Design review of the part built by this model. Coordinates are the model's own, in mm. A direction names the side the tool comes from. Give positions to 0.01 mm unless a question says otherwise; leave off trailing zeros. Write each loop counter-clockwise with the first axis right and the second up, starting at its lowest first coordinate (ties: lowest second). Pieces come first, ordered by that corner, then holes. Notation, with made-up numbers: (-19, 12.5) -> (37, 12.5) arc R38 cw to (37, 50.5) -> close; hole circle Ø9 at (52.25, -13.75). An arc over 180 degrees is marked (long way). Answer as a JSON object with one key per item and string values.
```python
from build123d import *

# Parameters (mm, degrees)
SKETCH_R        = 55
PAD_DEPTH       = 40
PAD_DEPTH_BACK  = 20
POCKET_DEPTH    = 42
POCKET001_DEPTH = 16
SKETCH004_R     = 67.5
SKETCH004_R_2   = 58
POCKET002_DEPTH = 0.7
POCKET003_DEPTH = 0.7
SKETCH006_R     = 1.4
POCKET004_DEPTH = 35
SKETCH007_R     = 1.9
POCKET005_DEPTH = 20
FILLET_R        = 5
FILLET001_R     = 5
FILLET002_R     = 5
FILLET003_R     = 5
CHAMFER_SIZE    = 2
CHAMFER001_SIZE = 1


with BuildPart() as part:
    # Sketch → Pad (new body, two sides)
    with BuildSketch(Plane.XZ) as pad_sk:
        with BuildLine():
            Line((-120, 75), (0, 75))
            ThreePointArc((-74.66808, -7.048245), (55.468993, -50.479608), (0, 75))
            ThreePointArc((-74.66808, -7.048245), (-83.30852, 13.959176), (-102.203647, 26.566441))
            ThreePointArc((-120, 50.506104), (-115.063539, 35.591198), (-102.203647, 26.566441))
            Line((-120, 75), (-120, 50.506104))
        make_face()
        Circle(SKETCH_R, mode=Mode.SUBTRACT)
    extrude(amount=PAD_DEPTH)
    extrude(pad_sk.sketch, amount=-PAD_DEPTH_BACK)

    # Sketch001 (on Face7 of Pad) → Pocket (cut)
    with BuildSketch(Plane(origin=(0, 20, 0), x_dir=(1, 0, 0), z_dir=(0, 1, 0))):
        with BuildLine():
            Line((46.551104, -18.140074), (74.636799, -51.611301))
            ThreePointArc((74.636799, -51.611301), (27.033088, 86.623267), (-90.743475, 0))
            Line((-211.758942, -108.831918), (-90.743475, 0))
            Line((-62.856731, -108.831918), (-211.758942, -108.831918))
            Line((-42.167317, -48.745498), (-62.856731, -108.831918))
            Line((9.780971, -48.993879), (-42.167317, -48.745498))
            Line((46.551104, -18.140074), (9.780971, -48.993879))
        make_face()
    extrude(amount=-POCKET_DEPTH, mode=Mode.SUBTRACT)

    # Sketch003 (on Face2 of Pocket) → Pocket001 (cut)
    with BuildSketch(Plane(origin=(0, -22, 0), x_dir=(1, 0, 0), z_dir=(0, 1, 0))):
        with BuildLine():
            ThreePointArc((0, -70), (66.404243, -22.146705), (42.018147, 55.986385))
            Line((42.018147, 55.986385), (62.226624, 86.16832))
            Line((62.226624, 86.16832), (-170.809082, 86.16832))
            Line((-170.809082, 86.16832), (-170.809082, -70))
            Line((-170.809082, -70), (0, -70))
        make_face()
    extrude(amount=-POCKET001_DEPTH, mode=Mode.SUBTRACT)

    # Sketch004 → Pocket002 (cut)
    with BuildSketch(Plane(origin=(0, -38, 0), x_dir=(-1, 0, 0), z_dir=(0, 1, 0))):
        Circle(SKETCH004_R)
        Circle(SKETCH004_R_2, mode=Mode.SUBTRACT)
    extrude(amount=-POCKET002_DEPTH, mode=Mode.SUBTRACT)

    # Sketch005 (on Face14 of Pocket002) → Pocket003 (cut)
    with BuildSketch(Plane(origin=(0, -38, 0), x_dir=(1, 0, 0), z_dir=(0, 1, 0))):
        Polygon((-1.938341, -67.163612), (-28.325365, -52.55386), (-167.517487, -52.55386), (-166.878586, -67.163612), align=None)
        Polygon((12.572289, 63.526501), (-92.206108, 90.359993), (-139.164734, 46.595844), align=None)
    extrude(amount=-POCKET003_DEPTH, mode=Mode.SUBTRACT)

    # Sketch006 (on Face4 of Pocket003) → Pocket004 (cut)
    with BuildSketch(Plane(origin=(0, 20, 0), x_dir=(1, 0, 0), z_dir=(0, 1, 0))):
        with Locations((-38.002514, -53.753925)):
            Circle(SKETCH006_R)
        with Locations((-43.871658, -69.918114)):
            Circle(SKETCH006_R)
        with Locations((-1.248232, -65.011124)):
            Circle(SKETCH006_R)
        with Locations((26.37031, -58.932541)):
            Circle(SKETCH006_R)
        with Locations((50.759274, -31.119787)):
            Circle(SKETCH006_R)
        with Locations((57.686783, -39.586739)):
            Circle(SKETCH006_R)
    extrude(amount=-POCKET004_DEPTH, mode=Mode.SUBTRACT)

    # Sketch007 (on Face4 of Pocket004) → Pocket005 (cut)
    with BuildSketch(Plane(origin=(0, 20, 0), x_dir=(1, 0, 0), z_dir=(0, 1, 0))):
        with Locations((-38.002514, -53.753925)):
            Circle(SKETCH007_R)
        with Locations((-43.871658, -69.918114)):
            Circle(SKETCH007_R)
        with Locations((-1.248232, -65.011124)):
            Circle(SKETCH007_R)
        with Locations((26.37031, -58.932541)):
            Circle(SKETCH007_R)
        with Locations((50.759274, -31.119787)):
            Circle(SKETCH007_R)
        with Locations((57.686783, -39.586739)):
            Circle(SKETCH007_R)
    extrude(amount=-POCKET005_DEPTH, mode=Mode.SUBTRACT)

    # Fillet
    fillet_edges = [part.edges().sort_by_distance(p)[0] for p in [
        (-50.346648, -22, 72.5),
    ]]
    fillet(fillet_edges, radius=FILLET_R)

    # Fillet001
    fillet001_edges = [part.edges().sort_by_distance(p)[0] for p in [
        (-120, -22, 72.5),
    ]]
    fillet(fillet001_edges, radius=FILLET001_R)

    # Fillet002
    fillet002_edges = [part.edges().sort_by_distance(p)[0] for p in [
        (62.35606, -22, 36.975687),
    ]]
    fillet(fillet002_edges, radius=FILLET002_R)

    # Fillet003
    fillet003_edges = [part.edges().sort_by_distance(p)[0] for p in [
        (43.410932, -22, -58.066548),
        (43.410932, -38, -58.066548),
    ]]
    fillet(fillet003_edges, radius=FILLET003_R)

    # Chamfer
    chamfer_edges = [part.edges().sort_by_distance(p)[0] for p in [
        (-46.687392, 20, 61.872749),
        (57.127061, 20, 30.744008),
    ]]
    chamfer(chamfer_edges, length=CHAMFER_SIZE)

    # Chamfer001
    chamfer001_edges = [part.edges().sort_by_distance(p)[0] for p in [
        (-60, -40, 75),
        (55.468993, -40, -50.479608),
        (-83.30852, -40, 13.959176),
        (-115.063539, -40, 35.591198),
        (-120, -40, 62.753052),
        (-55, -40, 0),
    ]]
    chamfer(chamfer001_edges, length=CHAMFER001_SIZE)


solid = part.part
```
(1) For line 1 along Z through (x, y) = (0, -38.35); line 2 along Y through (x, z) = (24, 64); line 3 along Y through (x, z) = (48, 42), list the stretches that pass through material, from the lowest coordinate up.
Here are the results:
{"line 1": "z = -75 to -67.5, -58 to -55, 55 to 58, 67.5 to 75", "line 2": "y = -40 to -38, -22 to 20", "line 3": "y = -40 to -38.7, -22 to 20"}
(2) For faces 1 (the flat face through (21, -38, 51)), 2 (the cylindrical face through (26.12, 10.14, 57.05)), 3 (the flat face through (43.391, -29.958, -58.037)), 4 (the flat face through (-85, -22, 72)), list the 3-axis set-ups (+Z, -Z, +X, -X, +Y, -Y) from which the entire face can be reached by the end or side of a thin tool; tool diameter is ignored.
Here are the results:
{"face 1": "-X", "face 2": "+Y", "face 3": "-Z, -X, +Y", "face 4": "+Z, -Z, -X, +Y"}
(3) We need section C-C, the plane y = -24.5. State the section outline as (x, z) points, then the cut area to 3 significant figures.
Here are the results:
{"outline": "(-119.33, 70) -> (0, 70) arc R70 cw to (42.55, -55.58) -> (45.34, -59.74) arc R75 ccw to (0, 75) -> (-119.33, 75) -> close", "area": "1,500 mm²"}
(4) We need section A-A, the plane y = 6. State the section outline as (x, z) points.
Here are the results:
{"outline": "(-51.21, 75) -> (-42.17, 48.75) -> (-25.32, 48.83) arc R55 cw to (50.19, 22.48) -> (64.06, 39.01) arc R75 ccw to (0, 75) -> close; hole circle Ø3.8 at (-43.87, 69.92); hole circle Ø3.8 at (-38, 53.75); hole circle Ø3.8 at (-1.25, 65.01); hole circle Ø3.8 at (26.37, 58.93); hole circle Ø3.8 at (50.76, 31.12); hole circle Ø3.8 at (57.69, 39.59)"}
(5) We need section B-B, the plane y = -11.5. State the section outline as (x, z) points, then the cut area to 3 significant figures.
Here are the results:
{"outline": "(-51.21, 75) -> (-42.17, 48.75) -> (-25.32, 48.83) arc R55 cw to (50.19, 22.48) -> (64.06, 39.01) arc R75 ccw to (0, 75) -> close; hole circle Ø2.8 at (-43.87, 69.92); hole circle Ø2.8 at (-38, 53.75); hole circle Ø2.8 at (-1.25, 65.01); hole circle Ø2.8 at (26.37, 58.93); hole circle Ø2.8 at (50.76, 31.12); hole circle Ø2.8 at (57.69, 39.59)", "area": "2,480 mm²"}
(6) The part is to be moulded in two halves that separate along Z. For faces 5 (the cylindrical face through (-51.991, -20.496, 72.896)), 6 (the flat face through (-51, -40, 28)), 7 (the flat face through (-48, -16, 75)), 8 (the cylindrical face through (-1.496, 10.14, 63.127)), say which applies: +Z half, -Z half, draft (parallel to the pull), parting line (faces both ways), or undercut.
Here are the results:
{"face 5": "-Z half", "face 6": "draft", "face 7": "+Z half", "face 8": "undercut"}
(7) Clearance check with flat-ended pins moving along their axes: pin 1 (4 mm diameter, centred on x = -100, z = 27.5, fed in from +Y); pin 2 (5 mm diameter, centred on x = 0, y = -6.5, fed in from -Z); pin 3 (10 mm diameter, centred on y = -12.5, z = 39.5, fed in from -X). State where each tip first meets the part, or that it passes through.
Here are the results:
{"pin 1": "stops at y = -38", "pin 2": "stops at z = 54.94", "pin 3": "stops at x = 32.32"}
